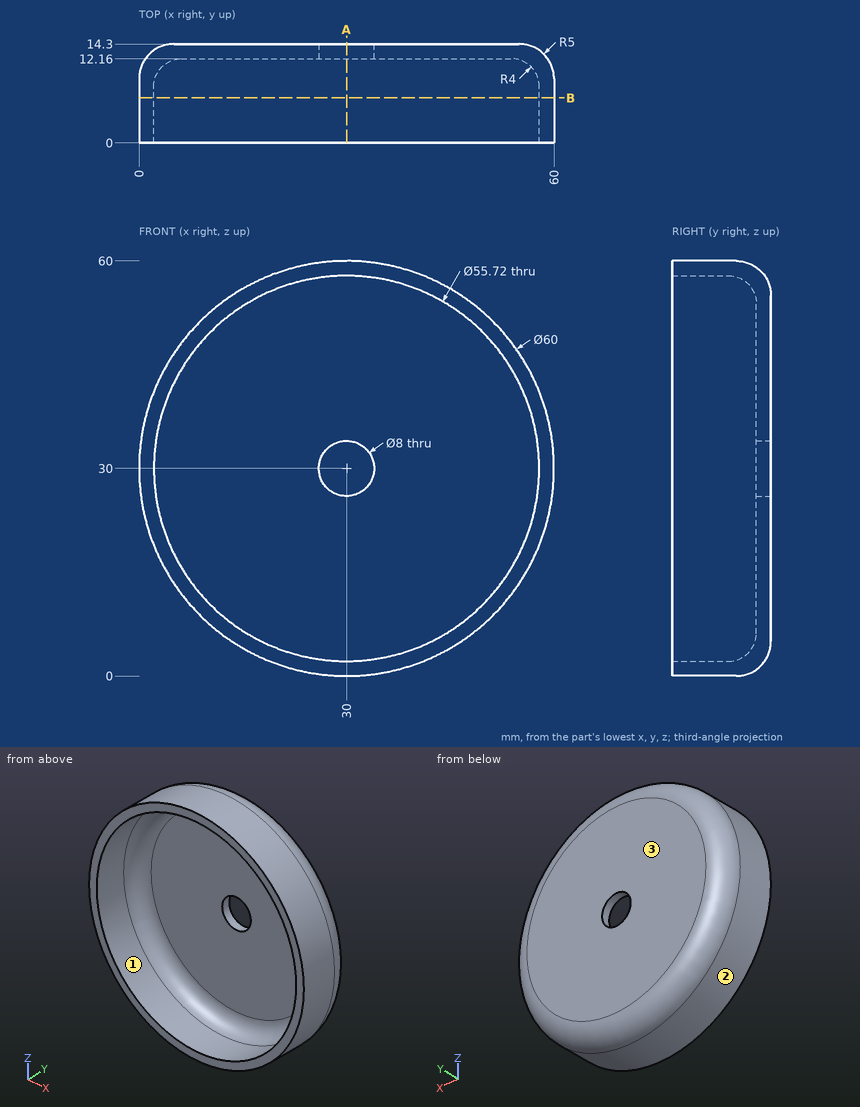
Geometry: see drawing. Coordinates: mm, zero at the bounding-box minimum. Coordinates: 2 decimals unless noted, no trailing zeros. Loops run counter-clockwise (first coordinate to the right, second up) from the corner with the lowest first, then second, coordinate; pieces in that order, holes last. Notation, with made-up numbers: (73.5, 1.25) - (113.5, 1.25) arc R32 cw to (113.5, 27.25) - close; hole circle Ø2 at (-8, -15.75). An arc over 180 degrees is marked (long way). Put each result on its own line as item: value. Start each with the question number.
Q1. Line query: line 1 (Z direction, x = 30, y = 3.75); line 2 (Y direction, x = 20, z = 23); line 3 (Z direction, x = 17, y = 3.5). Output: solid intervals per line, ascending.
Q2. Pin query (flat end, axial travel): pin 1 Ø4 at (y, z) = (4.5, 26.5) entering from -X; pin 2 Ø9 at (x, z) = (30, 30) entering from -Y; pin 3 Ø3 at (x, y) = (48, 3.5) entering from +Z. Return the tip coordinate at first contact, or that it passes through.
Q3. Cut plane A-A, the plane x = 30. Return loops of the section in (y, z), and give its area (3 significant figures).
Q4. Pull-direction query (X, two-part tool) for the marked faces 1, 2 and 3; classes: released by +X, released by -X, zero draft, split by the parting line, or undercut.
Q5. Cut plane B-B, the plane y = 6.5. Return loops of the section in (x, z).
Filled sheet:
1. line 1: 0 to 2.14, 57.86 to 60
1. line 2: 12.16 to 14.3
1. line 3: 2.96 to 5.36, 54.64 to 57.04
2. pin 1: x = 0.04
2. pin 2: y = 12.16
2. pin 3: z = 55.05
3. outline: (0, 0) - (9.3, 0) arc R5 ccw to (14.3, 5) - (14.3, 26) - (12.16, 26) - (12.16, 6.14) arc R4 cw to (8.16, 2.14) - (0, 2.14) - close; (0, 57.86) - (8.16, 57.86) arc R4 cw to (12.16, 53.86) - (12.16, 34) - (14.3, 34) - (14.3, 55) arc R5 ccw to (9.3, 60) - (0, 60) - close
3. area: 159 mm²
4. face 1: undercut
4. face 2: split by the parting line
4. face 3: zero draft
5. outline: circle Ø60 at (30, 30); hole circle Ø55.72 at (30, 30)
